Model file for the job. Use its own axes, mm. A direction names the side the tool comes from. Round coordinates to 2 decimals unless told otherwise and drop trailing zeros. Order: outer loops, then holes, each group sorted by start corner. A loop starts at its lowest first (then second) coordinate and runs counter-clockwise, first axis right, second up. Notation, with made-up numbers: (-8.5, 21.25) -> (-0.5, 21.25) arc R27 cw to (-0.5, 41.25) -> close; hole circle Ø9 at (-22.5, -19.75). An arc over 180 degrees is marked (long way). Answer as CSV lines item,"result".
```python
from build123d import *

# Parameters (mm, degrees)
SKETCH1_W           = 38
SKETCH1_H           = 40
SKETCH1_R           = 4.15
BOSS_EXTRUDE1_DEPTH = 5
FILLET1_R           = 6
SKETCH2_W           = 9.5
SKETCH2_H           = 4
BOSS_EXTRUDE2_DEPTH = 4
CHAMFER1_SIZE       = 2


with BuildPart() as part:
    # Sketch1 → Boss-Extrude1 (new body, symmetric)
    with BuildSketch(Plane.XY):
        Rectangle(SKETCH1_W, SKETCH1_H)
        Circle(SKETCH1_R, mode=Mode.SUBTRACT)
    extrude(amount=BOSS_EXTRUDE1_DEPTH, both=True)

    # Fillet1
    fillet1_edges = [part.edges().sort_by_distance(p)[0] for p in [
        (19, -20, 0),
        (-19, -20, 0),
        (-19, 20, 0),
        (19, 20, 0),
    ]]
    fillet(fillet1_edges, radius=FILLET1_R)

    # Sketch2 → Boss-Extrude2 (add)
    with BuildSketch(Plane.XY.offset(5)):
        with Locations((0, 18)):
            Rectangle(SKETCH2_W, SKETCH2_H)
        with Locations((0, -18)):
            Rectangle(SKETCH2_W, SKETCH2_H)
    extrude(amount=BOSS_EXTRUDE2_DEPTH)

    # Chamfer1
    chamfer1_edges = [part.edges().sort_by_distance(p)[0] for p in [
        (4.75, 18, 9),
        (-4.75, 18, 9),
        (-4.75, -18, 9),
        (4.75, -18, 9),
    ]]
    chamfer(chamfer1_edges, length=CHAMFER1_SIZE)


solid = part.part
```
Q1. Tool access for faces 1 (the flat face through (-4.75, 18, 6)), 2 (the flat face through (4.75, -18, 6)), 3 (the flat face through (0, 16, 7)), 4 (the flat face through (-19, 0, 0)), 5 (the cylindrical face through (17.289, 18.196, -0.07)): list every direction of +Z, -Z, +X, -X, +Y, -Y with a clear straight run to the whole face (end or side of a thin tool).
Checks:
face 1,"+Z, -X, +Y, -Y"
face 2,"+Z, +X, +Y, -Y"
face 3,"+Z, +X, -X"
face 4,"+Z, -Z, -X, +Y, -Y"
face 5,"+Z, -Z, +X, +Y"
Q2. Saw through at B-B (x = 0). Write the cut outline in (y, z), plus the area to 3 significant figures.
Checks:
outline,"(-20, -5) -> (-4.15, -5) -> (-4.15, 5) -> (-16, 5) -> (-16, 9) -> (-20, 9) -> close; (4.15, -5) -> (20, -5) -> (20, 9) -> (16, 9) -> (16, 5) -> (4.15, 5) -> close"
area,"349 mm²"
Q3. Mould opens along Y. For faces 6 (the flat face through (0, -16, 7)), 7 (the cylindrical face through (17.289, -18.196, 0.07)), 8 (the flat face through (-3.74, -18.03, 8.01)) say: +Y half, -Y half, draft (parallel to the pull), parting line (faces both ways), or undercut.
Checks:
face 6,"undercut"
face 7,"-Y half"
face 8,"draft"
Q4. Wall check: L1, parallel to Y at x = 0, z = -2; L2, parallel to Z at x = -14, y = 8; L3, parallel to Y at x = -1, z = 2.25. Give the ranges that are in metal, low to high. Write a range as [from, to].
Checks:
L1,"[-20, -4.15], [4.15, 20]"
L2,"[-5, 5]"
L3,"[-20, -4.03], [4.03, 20]"
Q5. Saw through at D-D (x = 9.5). Write the cut outline in (y, z), plus the area to 3 significant figures.
Checks:
outline,"(-20, -5) -> (20, -5) -> (20, 5) -> (-20, 5) -> close"
area,"400 mm²"
Q6. Saw through at A-A (y = 0). Write the cut outline in (x, z).
Checks:
outline,"(-19, -5) -> (-4.15, -5) -> (-4.15, 5) -> (-19, 5) -> close; (4.15, -5) -> (19, -5) -> (19, 5) -> (4.15, 5) -> close"
Q7. Saw through at C-C (z = -3.5). Write the cut outline in (x, y).
Checks:
outline,"(-19, -14) arc R6 ccw to (-13, -20) -> (13, -20) arc R6 ccw to (19, -14) -> (19, 14) arc R6 ccw to (13, 20) -> (-13, 20) arc R6 ccw to (-19, 14) -> close; hole circle Ø8.3 at (0, 0)"
Q8. Flat gauge pins, fed straight in: pin 1 (6 mm diameter, centred on x = -12.5, y = -14, fed in from +Z); pin 2 (2 mm diameter, centred on y = 17.5, z = 6.5, fed in from -X); pin 3 (0.6 mm diameter, centred on y = -19, z = 6, fed in from +X); pin 4 (5 mm diameter, centred on y = 4.5, z = 6.5, fed in from -X). Where does each tip first touch, or does it go through?
Checks:
pin 1,"z = 5"
pin 2,"x = -4.75"
pin 3,"x = 4.75"
pin 4,"x = -19"
